```python
from build123d import *
from build123d.topology import SkipClean

# Parameters (mm, degrees)
SKETCH28_R           = 1.55
SKETCH28_R_2         = 13
SKETCH28_R_3         = 4.5
SKETCH28_W           = 10
SKETCH28_H           = 3
BOSS_EXTRUDE10_DEPTH = 5
SKETCH29_R           = 16
SKETCH29_R_2         = 8.2
BOSS_EXTRUDE11_DEPTH = 5


with BuildPart() as part:
    # Sketch28 → Boss-Extrude10 (new body)
    with BuildSketch(Plane(origin=(-32, 0, 0), x_dir=(0, 0, 1), z_dir=(0, -1, 0))):
        with BuildLine():
            Line((-25, 15), (25, 15))
            Line((25, 15), (25, 5))
            Line((25, 5), (16, -145))
            ThreePointArc((16, -145), (0, -161), (-16, -145))
            Line((-16, -145), (-25, 5))
            Line((-25, 5), (-25, 15))
        make_face()
        with Locations(Location((8, 8.5, 0), (0, 0, 180))):
            Circle(SKETCH28_R, mode=Mode.SUBTRACT)
        with Locations(Location((-8, 8.5, 0), (0, 0, 180))):
            Circle(SKETCH28_R, mode=Mode.SUBTRACT)
        with Locations(Location((16, 11.5, 0), (0, 0, 180))):
            Circle(SKETCH28_R, mode=Mode.SUBTRACT)
        with Locations(Location((-16, 11.5, 0), (0, 0, 180))):
            Circle(SKETCH28_R, mode=Mode.SUBTRACT)
        with Locations(Location((-15.5, -6, 0), (0, 0, 180))):
            Circle(SKETCH28_R, mode=Mode.SUBTRACT)
        with Locations(Location((15.5, -6, 0), (0, 0, 180))):
            Circle(SKETCH28_R, mode=Mode.SUBTRACT)
        with Locations(Location((0, -20.7, 0), (0, 0, 180))):
            Circle(SKETCH28_R_2, mode=Mode.SUBTRACT)
        with Locations(Location((0, -145, 0), (0, 0, 180))):
            Circle(SKETCH28_R_3, mode=Mode.SUBTRACT)
        with Locations((0, -4.5)):
            Rectangle(SKETCH28_W, SKETCH28_H, mode=Mode.SUBTRACT)
    extrude(amount=BOSS_EXTRUDE10_DEPTH)

    # Sketch29 → Boss-Extrude11 (add)
    with SkipClean():  # the faces are left unmerged after this step: merging them gives an invalid solid
        with BuildSketch(Plane.XZ.offset(5)):
            with Locations(Location((113, 0, 0), (0, 0, 270))):
                Circle(SKETCH29_R)
            with Locations(Location((113, 0, 0), (0, 0, 270))):
                Circle(SKETCH29_R_2, mode=Mode.SUBTRACT)
        extrude(amount=BOSS_EXTRUDE11_DEPTH)
    add(part.part.scale(1), mode=Mode.REPLACE)  # the faces are merged on a copy


solid = part.part
```
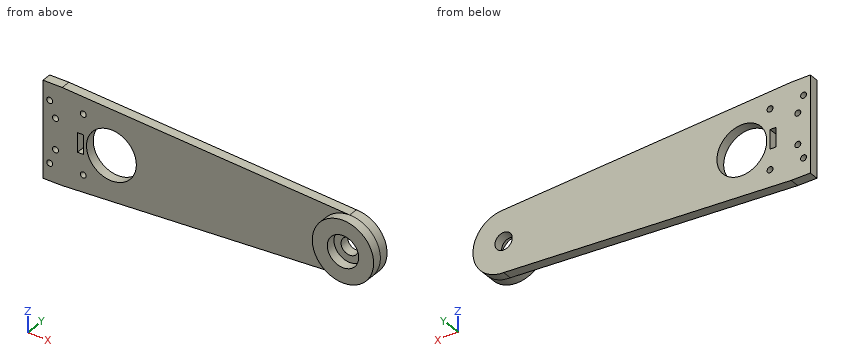
The model under review builds one solid part; all positions refer to its coordinate system, in mm. Give positions to 0.01 mm unless a question says otherwise; leave off trailing zeros. Write each loop counter-clockwise with the first axis right and the second up, starting at its lowest first coordinate (ties: lowest second). Pieces come first, ordered by that corner, then holes. Notation, with made-up numbers: M -28,32.25 L 18,32.25 A27 ccw 18,64.25 Z; hole C 22.25,2 d5. An arc over 180 degrees is marked long. Write each question's results on one line, items separated by ' | '. Start each with the question number.
1. For probe 1 along X at (y, z) = (-6.5, 0); probe 2 along X at (y, z) = (-3.5, 9); probe 3 along Y at (x, z) = (-26, -7), list the stretches that pass through material, from the lowest coordinate up. Write a range as [from, to].
2. We need section D-D (x = 100). Write out the cut boundary in (y, z), and give its area (3 significant figures).
3. We need section C-C (x = -11.3). Write out the cut boundary in (y, z).
4. Insertion check: pin 1 Ø3 at (x, z) = (-26, -15.5) entering from +Y; pin 2 Ø1 at (x, z) = (81, -5) entering from -Y; pin 3 Ø3 at (x, z) = (107.5, -14.5) entering from +Y; pin 4 Ø5 at (x, y) = (15.5, -3) entering from -Z. Each pin has a flat end and moves straight along its axis. Give the tip position at first contact, or say it passes through.
5. We need section A-A (y = -2). Count the separate pieces of the cut face and the enclosed holes in it, and give its area (3 significant figures).
6. We need section B-B (z = -3). Write out the cut boundary in (x, y), and give its area (3 significant figures).
Results found:
1) probe 1: x = [97, 104.8], [121.2, 129] | probe 2: x = [-47, -41.68], [-39.32, -20.68], [-1.92, 126.23] | probe 3: y = [-5, 0]
2) outline: M -10,-9.33 L -5,-9.33 L -5,-16.78 L 0,-16.78 L 0,16.78 L -5,16.78 L -5,9.33 L -10,9.33 Z | area: 261 mm^2
3) outline: M -5,-23.46 L 0,-23.46 L 0,-13 L -5,-13 Z; M -5,13 L 0,13 L 0,23.46 L -5,23.46 Z
4) pin 1: passes through | pin 2: stops at y = -5 | pin 3: stops at y = 0 | pin 4: stops at z = -22
5) separate pieces: 1 | enclosed holes: 9 | area: 6,380 mm^2
6) outline: M -47,-5 L -29,-5 L -29,0 L -47,0 Z; M -26,-5 L -23.95,-5 L -23.95,0 L -26,0 Z; M 1.35,-5 L 97.28,-5 L 97.28,-10 L 105.37,-10 L 105.37,-5 L 109.65,-5 L 109.65,0 L 1.35,0 Z; M 116.35,-5 L 120.63,-5 L 120.63,-10 L 128.72,-10 L 128.72,0 L 116.35,0 Z | area: 784 mm^2
